Verification items for the finished model (mm, model axes). Face numbers are marked on the shaded views. A direction names the side the tool comes from. Give positions to 0.01 mm unless a question says otherwise; leave off trailing zeros. Write each loop counter-clockwise with the first axis right and the second up, starting at its lowest first coordinate (ties: lowest second). Pieces come first, ordered by that corner, then holes. Notation, with made-up numbers: (-8.75, -35.5) -> (1.25, -35.5) arc R14 ccw to (1.25, -23.5) -> close; hole circle Ø5 at (69, 78). An arc over 180 degrees is marked (long way). Use one line per item in the form item = value. Start each with the question number.
(1) Section check D-D, the plane z = -3.75. Record the cut outline in (x, y).
(2) Section check A-A, the plane x = -18.5. Record the cut outline in (y, z).
(3) Release check for a two-part mould opening along X. For the marked faces 6, 7 and 8 record: pulls with the +X half, pulls with the -X half, needs draft (parallel to the pull), parting line crosses it, or undercut.
(4) Scan lines: L1, parallel to X at y = 5, z = 0; L2, parallel to X at y = 9.9, z = 0; L3, parallel to Y at x = 3.75, z = 0. Record each from-to range of solid material in increasing order.
(5) Depth check by flat-ended pin: pin 1 Ø1.5 at (x, y) = (10.5, 2.5) entering from +Z; pin 2 Ø1 at (x, z) = (5.5, 4) entering from -Y; pin 3 Ø3 at (x, z) = (-11.5, -0.5) entering from -Y. Enter the tip coordinate at first touch or a pass-through.
(6) Section check C-C, the plane x = 11.5. Record the cut outline in (y, z), plus the area to 3 significant figures.
(7) Set-up check for the marked faces 1, 2, 3, 4 and 5: record each of +Z, -Z, +X, -X, +Y, -Y from which the full face is reachable in a straight line by a thin tool's end or side.
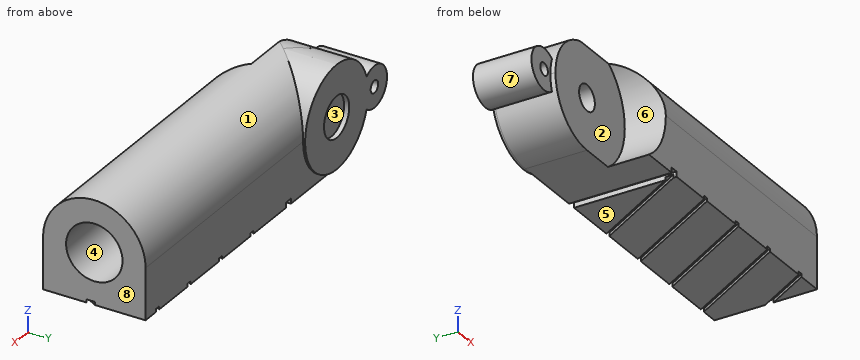
from build123d import *

# Parameters (mm, degrees)
SKETCH_1_W          = 35
SKETCH_1_H          = 10
EXTRUDE_1_DEPTH     = 10
FILLET_1_R          = 5
SKETCH_3_R          = 6
CUT_EXTRUDE_1_DEPTH = 4
SKETCH_7_R          = 5
EXTRUDE_4_DEPTH     = 0.2
SKETCH_8_R          = 2
CUT_EXTRUDE_3_DEPTH = 0.5
FILLET_3_R          = 5
SKETCH_10_R         = 2
EXTRUDE_5_DEPTH     = 5.7
SKETCH_11_R         = 0.6
CUT_EXTRUDE_4_DEPTH = 24.436936812
SKETCH_12_R         = 2.75
CUT_EXTRUDE_5_DEPTH = 23
SKETCH_6_R          = 1.25
CUT_EXTRUDE_6_DEPTH = 4
FILLET_4_R          = 1
SKETCH_13_W         = 0.8
SKETCH_13_H         = 10
CUT_EXTRUDE_7_DEPTH = 0.5
CUT_EXTRUDE_8_DEPTH = 0.3


# Some blends are built 0.0001 mm under size
with BuildPart() as part:
    # 草图1 → 凸台-拉伸1 (new body)
    with BuildSketch(Plane(origin=(0, 0, 0), x_dir=(1, 0, 0), z_dir=(0, 1, 0))):
        Rectangle(SKETCH_1_W, SKETCH_1_H)
    extrude(amount=EXTRUDE_1_DEPTH)

    # 圆角1
    fillet_1_edges = [part.edges().sort_by_distance(p)[0] for p in [
        (-17.5, 5, 5),
        (-17.5, 5, -5),
    ]]
    fillet(fillet_1_edges, radius=FILLET_1_R - 0.0001)  # a hair under: the kernel refuses the full size

    # 草图3 → 切除-拉伸1 (cut)
    with BuildSketch(Plane.XZ):
        with Locations((-12.5, 0)):
            Circle(SKETCH_3_R)
    extrude(amount=-CUT_EXTRUDE_1_DEPTH, mode=Mode.SUBTRACT)

    # 草图7 → 凸台-拉伸4 (add)
    with BuildSketch(Plane(origin=(0, 10, 0), x_dir=(1, 0, 0), z_dir=(0, 1, 0))):
        with Locations(Location((-12.5, 0, 0), (0, 0, 270))):
            Circle(SKETCH_7_R)
    extrude(amount=EXTRUDE_4_DEPTH)

    # 草图8 → 切除-拉伸3 (cut)
    with BuildSketch(Plane(origin=(0, 10.2, 0), x_dir=(1, 0, 0), z_dir=(0, 1, 0))):
        with Locations(Location((-12.5, 0, 0), (0, 0, 270))):
            Circle(SKETCH_8_R)
    extrude(amount=-CUT_EXTRUDE_3_DEPTH, mode=Mode.SUBTRACT)

    # 圆角3
    # the kernel refuses this fillet: 5 mm, written as the material it takes off along each edge
    with BuildSketch(Plane(origin=(30, 0, 5), x_dir=(0, 1, 0), z_dir=(-1, 0, 0))) as fillet_3_piece_1:
        with BuildLine():
            CenterArc((FILLET_3_R, FILLET_3_R), FILLET_3_R, 180, 90)
            Line((0, FILLET_3_R), (0, 0))
            Line((0, 0), (FILLET_3_R, 0))
        make_face()
    extrude(amount=51.68337521, mode=Mode.SUBTRACT)
    with BuildSketch(Plane(origin=(30, 10, 5), x_dir=(0, -1, 0), z_dir=(-1, 0, 0))) as fillet_3_piece_2_section:
        with BuildLine():
            CenterArc((FILLET_3_R, -FILLET_3_R), FILLET_3_R, 90, 90)
            Line((0, -FILLET_3_R), (0, 0))
            Line((0, 0), (FILLET_3_R, 0))
        make_face()
    fillet_3_piece_2 = extrude(amount=55, mode=Mode.PRIVATE)
    fillet_3_piece_2 = fillet_3_piece_2 - Plane(origin=(-12.5, 8.593554342, 0), x_dir=(0, 0, 1), z_dir=(0, -1, 0)) * Cylinder(5, 130, mode=Mode.PRIVATE)
    add(fillet_3_piece_2, mode=Mode.SUBTRACT)

    # 草图10 → 凸台-拉伸5 (add)
    with BuildSketch(Plane(origin=(0, 10.2, 0), x_dir=(1, 0, 0), z_dir=(0, 1, 0))):
        with Locations((-18.5, 0)):
            Circle(SKETCH_10_R)
    extrude(amount=-EXTRUDE_5_DEPTH)

    # 草图11 → 切除-拉伸4 (cut, through all)
    with BuildSketch(Plane(origin=(0, 10.2, 0), x_dir=(1, 0, 0), z_dir=(0, 1, 0))):
        with Locations(Location((-18.5, 0, 0), (0, 0, 270))):
            Circle(SKETCH_11_R)
    extrude(amount=-CUT_EXTRUDE_4_DEPTH, mode=Mode.SUBTRACT)

    # 草图12 → 切除-拉伸5 (cut)
    with BuildSketch(Plane(origin=(17.5, 0, 0), x_dir=(0, 0, -1), z_dir=(1, 0, 0))):
        with Locations((0, 5)):
            Circle(SKETCH_12_R)
    extrude(amount=-CUT_EXTRUDE_5_DEPTH, mode=Mode.SUBTRACT)

    # 草图6 → 切除-拉伸6 (cut)
    with BuildSketch(Plane.XZ.offset(-4)):
        with Locations(Location((-12.5, 0, 0), (0, 0, 270))):
            Circle(SKETCH_6_R)
    extrude(amount=-CUT_EXTRUDE_6_DEPTH, mode=Mode.SUBTRACT)

    # 圆角4
    fillet_4_edges = [part.edges().sort_by_distance(p)[0] for p in [
        (-5.5, 5, 2.75),
    ]]
    fillet(fillet_4_edges, radius=FILLET_4_R)

    # 草图13 → 切除-拉伸7 (cut)
    with BuildSketch(Plane(origin=(0, 0, -5), x_dir=(-1, 0, 0), z_dir=(0, 0, -1))):
        with Locations((5.18337521, 5)):
            Rectangle(SKETCH_13_W, SKETCH_13_H)
    extrude(amount=-CUT_EXTRUDE_7_DEPTH, mode=Mode.SUBTRACT)

    # 草图14 → 切除-拉伸8 (cut)
    with BuildSketch(Plane(origin=(0, 0, -5), x_dir=(-1, 0, 0), z_dir=(0, 0, -1))):
        Polygon((-10.031126924, -7.880483284), (-20.59026218, 10.408475463), (-20.936672342, 10.208475463), (-10.377537086, -8.080483284), align=None)
        Polygon((-5.031126924, -7.880483284), (-15.59026218, 10.408475463), (-15.936672342, 10.208475463), (-5.377537086, -8.080483284), align=None)
        Polygon((-0.031126924, -7.880483284), (-10.59026218, 10.408475463), (-10.936672342, 10.208475463), (-0.377537086, -8.080483284), align=None)
        Polygon((4.968873076, -7.880483284), (-5.59026218, 10.408475463), (-5.936672342, 10.208475463), (4.622462914, -8.080483284), align=None)
        Polygon((9.968873076, -7.880483284), (-0.59026218, 10.408475463), (-0.936672342, 10.208475463), (9.622462914, -8.080483284), align=None)
    extrude(amount=-CUT_EXTRUDE_8_DEPTH, mode=Mode.SUBTRACT)


solid = part.part
Completed:
q1.outline = (-15.81, 4) -> (-7.82, 4) -> (-7.82, 0) -> (17.5, 0) -> (17.5, 10) -> (-9.19, 10) -> (-9.19, 10.2) -> (-15.81, 10.2) -> close
q2.outline = (4.5, -2) -> (10.2, -2) -> (10.2, -0.6) -> (4.5, -0.6) -> close; (4.5, 0.6) -> (10.2, 0.6) -> (10.2, 2) -> (4.5, 2) -> close
q3.face_6 = pulls with the -X half
q3.face_7 = undercut
q3.face_8 = pulls with the +X half
q4.L1 = -20.5 to -19.1, -17.9 to -13.75, -11.25 to -5.5
q4.L2 = -20.5 to -19.1, -17.9 to -14.5, -10.5 to 17.5
q4.L3 = 0 to 2.25, 7.75 to 10
q5.pin_1 = 4.68
q5.pin_2 = 1.43
q5.pin_3 = 4
q6.outline = (0, -5) -> (2.52, -5) -> (2.52, -4.7) -> (3.32, -4.7) -> (3.32, -5) -> (10, -5) -> (10, 0) arc R5 ccw to (0, 0) -> close; hole circle Ø5.5 at (5, 0)
q6.area = 65.3 mm²
q7.face_1 = +Z, +X
q7.face_2 = -X, -Y
q7.face_3 = +Y
q7.face_4 = +X
q7.face_5 = -Z, +X, -X, +Y, -Y
